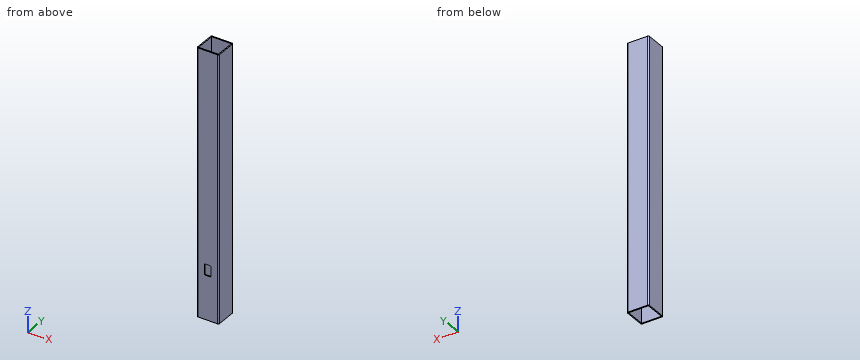
```python
from build123d import *

# Parameters (mm, degrees)
F0_W     = 90
F0_H     = 90
F1_DEPTH = 1212
F3_DEPTH = 4


with BuildPart() as f1:
    # F0 (on Top) → F1 (new body)
    with BuildSketch(Plane.XY):
        with BuildLine():
            ThreePointArc((50, 45), (48.535534, 48.535534), (45, 50))
            Line((45, 50), (-45, 50))
            ThreePointArc((-45, 50), (-48.535534, 48.535534), (-50, 45))
            Line((-50, 45), (-50, -45))
            ThreePointArc((-50, -45), (-48.535534, -48.535534), (-45, -50))
            Line((-45, -50), (45, -50))
            ThreePointArc((45, -50), (48.535534, -48.535534), (50, -45))
            Line((50, -45), (50, 45))
        make_face()
        Rectangle(F0_W, F0_H, mode=Mode.SUBTRACT)
    extrude(amount=F1_DEPTH)

    # F2 (on face) → F3 (cut)
    with BuildSketch(Plane.XZ.offset(50)):
        with BuildLine():
            ThreePointArc((-15, 205), (-13.535534, 201.464466), (-10, 200))
            Line((-10, 200), (10, 200))
            ThreePointArc((10, 200), (13.535534, 201.464466), (15, 205))
            Line((15, 205), (15, 245))
            ThreePointArc((15, 245), (13.535534, 248.535534), (10, 250))
            Line((10, 250), (-10, 250))
            ThreePointArc((-10, 250), (-13.535534, 248.535534), (-15, 245))
            Line((-15, 245), (-15, 205))
        make_face()
    extrude(amount=-F3_DEPTH, mode=Mode.SUBTRACT)


solid = f1.part
```
Check sheet for the modelled part. Datum: model origin and axes. Units: mm. Round coordinates to 2 decimals unless told otherwise and drop trailing zeros. Order: outer loops, then holes, each group sorted by start corner. A loop starts at its lowest first (then second) coordinate and runs counter-clockwise, first axis right, second up. Notation, with made-up numbers: (-18, -23.75) -> (33, -23.75) arc R13 ccw to (33, -10.75) -> close; hole circle Ø10 at (30, 17). An arc over 180 degrees is marked (long way). Use CSV: the item, a comma, the result in double quotes.
(1) Depth check by flat-ended pin: pin 1 (1.2 mm diameter, centred on y = -49, z = 232, fed in from +X); pin 2 (4.5 mm diameter, centred on y = -48.5, z = 219.5, fed in from -X); pin 3 (15 mm diameter, centred on x = -6, z = 219, fed in from -Y). Enter the tip coordinate at first touch or a pass-through.
Worked out:
pin 1,"x = 48.67"
pin 2,"x = -49.84"
pin 3,"y = -46"
(2) Material ranges on line 1 along Y through (x, z) = (-35.5, 52), recorded low to high. Write a range as from..to.
Worked out:
line 1,"-50..-45, 45..50"
(3) Cross-section at C-C (z = 1089.5). Record the boundary of the cut face in (x, y), and give its area (3 significant figures).
Worked out:
outline,"(-50, -45) arc R5 ccw to (-45, -50) -> (45, -50) arc R5 ccw to (50, -45) -> (50, 45) arc R5 ccw to (45, 50) -> (-45, 50) arc R5 ccw to (-50, 45) -> close; hole (-45, -45) -> (45, -45) -> (45, 45) -> (-45, 45) -> close"
area,"1,880 mm²"
(4) Cross-section at A-A (x = -32.5). Record the boundary of the cut face in (y, z).
Worked out:
outline,"(-50, 0) -> (-45, 0) -> (-45, 1212) -> (-50, 1212) -> close; (45, 0) -> (50, 0) -> (50, 1212) -> (45, 1212) -> close"
